Geometry: final body of the model. Coordinates: model frame, mm. Face numbers are marked on the shaded views. A direction names the side the tool comes from. Coordinates: 2 decimals unless noted, no trailing zeros. Write each loop counter-clockwise with the first axis right and the second up, starting at its lowest first coordinate (ties: lowest second). Pieces come first, ordered by that corner, then holes. Notation, with made-up numbers: (73, 89) -> (88, 89) arc R11 cw to (88, 100) -> close; hole circle Ø7 at (22, 13.25). An arc over 180 degrees is marked (long way). One line per item, written item: value.
```python
from build123d import *

# Parameters (mm, degrees)
F0_W     = 50
F0_H     = 50
F1_DEPTH = 50
F3_R     = 16.4282141223
F4_DEPTH = 150
F5_R     = 6.4806520978
F6_DEPTH = 100


with BuildPart() as f1:
    # F0 (on Top) → F1 (new body)
    with BuildSketch(Plane.XY):
        with Locations((25, 25)):
            Rectangle(F0_W, F0_H)
    extrude(amount=F1_DEPTH)

    # F3 (on face) → F4 (join)
    with BuildSketch(Plane.XZ):
        with Locations((20.9893193096, 29.0806218982)):
            Circle(F3_R)
    extrude(amount=F4_DEPTH)

    # F5 (on face) → F6 (cut)
    with BuildSketch(Plane.XZ.offset(150)):
        with Locations((21.6495357454, 26.772018522)):
            Circle(F5_R)
    extrude(amount=-F6_DEPTH, mode=Mode.SUBTRACT)


solid = f1.part
```
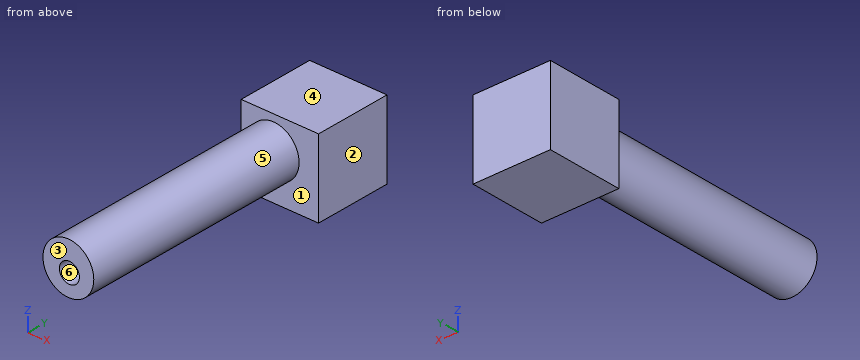
(1) Line query: line 1 (Y direction, x = 37, z = 8.5); line 2 (Z direction, x = 19, y = -141); line 3 (Z direction, x = 26.5, y = -107). Output: solid intervals per line, ascending. Write a range as [from, to].
Responses:
line 1: y = [0, 50]
line 2: z = [12.77, 20.86], [32.69, 45.39]
line 3: z = [13.6, 22.47], [31.07, 44.56]
(2) Pull-direction query (Z, two-part tool) for the marked faces 3, 4, 5 and 6; classes: released by +Z, released by -Z, zero draft, split by the parting line, or undercut.
Responses:
face 3: zero draft
face 4: released by +Z
face 5: split by the parting line
face 6: undercut
(3) Reachability of the marked faces 1 and 2 from +Z, -Z, +X, -X, +Y, -Y: full face, straight path, thin tool, end or side. Return the list, or none.
Responses:
face 1: -Y
face 2: +Z, -Z, +X, +Y, -Y
(4) Section C-C (y = -58). Return the cut outline in (x, z), then the cut area to 3 significant figures.
Responses:
outline: circle Ø32.86 at (20.99, 29.08); hole circle Ø12.96 at (21.65, 26.77)
area: 716 mm2
(5) First-contact query: pin 1 (15 mm diameter, centred on x = 21.65, z = 26.77, fed in from -Y); pin 2 (6 mm diameter, centred on y = -34.5, z = 42, fed in from -X); pin 3 (2 mm diameter, centred on y = -76.5, z = 41.5, fed in from -X); pin 4 (4 mm diameter, centred on x = 23.5, z = 27, fed in from -Y). Flat tips, straight axial feed; report the tip coordinate or a pass-through.
Responses:
pin 1: stops at y = -150
pin 2: stops at x = 7.89
pin 3: stops at x = 9.18
pin 4: stops at y = -50
(6) Section B-B (x = 22.5). Return the cut outline in (y, z), then the cut area to 3 significant figures.
Responses:
outline: (-150, 12.72) -> (0, 12.72) -> (0, 0) -> (50, 0) -> (50, 50) -> (0, 50) -> (0, 45.44) -> (-150, 45.44) -> (-150, 33.2) -> (-50, 33.2) -> (-50, 20.35) -> (-150, 20.35) -> close
area: 6,120 mm2
(7) Section A-A (z = 22.5). Return the cut outline in (x, y).
Responses:
outline: (0, 0) -> (5.94, 0) -> (5.94, -150) -> (16.78, -150) -> (16.78, -50) -> (26.52, -50) -> (26.52, -150) -> (36.04, -150) -> (36.04, 0) -> (50, 0) -> (50, 50) -> (0, 50) -> close
(8) Section D-D (z = 10). Return the cut outline in (x, y).
Responses:
outline: (0, 0) -> (50, 0) -> (50, 50) -> (0, 50) -> close
